from build123d import *

# Parameters (mm, degrees)
SKETCH3_W           = 40
SKETCH3_H           = 40
SKETCH3_R           = 5
SKETCH3_R_2         = 2.4
BOSS_EXTRUDE2_DEPTH = 3
BOSS_EXTRUDE3_DEPTH = 8
SKETCH6_W           = 2
SKETCH6_H           = 5
BOSS_EXTRUDE5_DEPTH = 5
SKETCH7_W           = 40
SKETCH7_H           = 6.5
CUT_EXTRUDE1_DEPTH  = 3
SKETCH8_W           = 40
SKETCH8_H           = 6.5
CUT_EXTRUDE2_DEPTH  = 3
CUT_EXTRUDE3_START  = -1
SKETCH5_W           = 5
SKETCH5_H           = 0.5
CUT_EXTRUDE3_DEPTH  = 6


with BuildPart() as part:
    # Sketch3 → Boss-Extrude2 (new body)
    with BuildSketch(Plane(origin=(0, 0, 0), x_dir=(1, 0, 0), z_dir=(0, 1, 0))):
        Rectangle(SKETCH3_W, SKETCH3_H)
        Circle(SKETCH3_R, mode=Mode.SUBTRACT)
        Circle(SKETCH3_R)
        Circle(SKETCH3_R_2, mode=Mode.SUBTRACT)
    extrude(amount=-BOSS_EXTRUDE2_DEPTH)

    # Sketch4 → Boss-Extrude3 (add)
    with BuildSketch(Plane.XZ.offset(3)):
        Polygon((20, -11.5), (0, -11.5), (-20, -11.5), (-20, -13.5), (20, -13.5), align=None)
        Polygon((-20, 11.5), (0, 11.5), (20, 11.5), (20, 13.5), (-20, 13.5), align=None)
    extrude(amount=BOSS_EXTRUDE3_DEPTH)

    # Sketch6 → Boss-Extrude5 (add)
    with BuildSketch(Plane.XZ.offset(3)):
        with Locations((19, 9)):
            Rectangle(SKETCH6_W, SKETCH6_H)
        with Locations((19, -9)):
            Rectangle(SKETCH6_W, SKETCH6_H)
        with Locations((-19, -9)):
            Rectangle(SKETCH6_W, SKETCH6_H)
        with Locations((-19, 9)):
            Rectangle(SKETCH6_W, SKETCH6_H)
    extrude(amount=BOSS_EXTRUDE5_DEPTH)

    # Sketch7 → Cut-Extrude1 (cut)
    with BuildSketch(Plane(origin=(0, -3, 0), x_dir=(-1, 0, 0), z_dir=(0, -1, 0))):
        with Locations((0, -16.75)):
            Rectangle(SKETCH7_W, SKETCH7_H)
    extrude(amount=-CUT_EXTRUDE1_DEPTH, mode=Mode.SUBTRACT)

    # Sketch8 → Cut-Extrude2 (cut)
    with BuildSketch(Plane.XZ.offset(3)):
        with Locations((0, -16.75)):
            Rectangle(SKETCH8_W, SKETCH8_H)
    extrude(amount=-CUT_EXTRUDE2_DEPTH, mode=Mode.SUBTRACT)

    # Sketch5 → Cut-Extrude3 (cut)
    with BuildSketch(Plane.XY.offset(-11.5).offset(CUT_EXTRUDE3_START)):
        Polygon((19, -7.5), (0, -7.5), (0, -8), (5, -8), (5, -8.5), (19, -8.5), align=None)
        Polygon((0, -8), (0, -7.5), (-19, -7.5), (-19, -8.5), (-5, -8.5), (-5, -8), align=None)
        with Locations((-2.5, -8.25)):
            Rectangle(SKETCH5_W, SKETCH5_H)
        with Locations((2.5, -8.25)):
            Rectangle(SKETCH5_W, SKETCH5_H)
    cut_extrude3 = extrude(amount=CUT_EXTRUDE3_DEPTH, mode=Mode.SUBTRACT)

    # Mirror2: Cut-Extrude3 across plane
    add(cut_extrude3.mirror(Plane.XY), mode=Mode.SUBTRACT)


solid = part.part
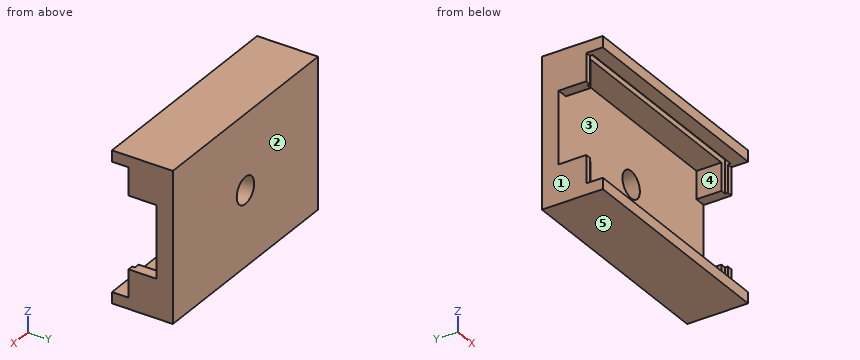
Read the model definition and answer for the solid it produces. Units are mm, in the model's axes. Face numbers are marked on the shaded views. A direction names the side the tool comes from. Coordinates: 2 decimals unless noted, no trailing zeros. Order: outer loops, then holes, each group sorted by start corner. A loop starts at its lowest first (then second) coordinate and runs counter-clockwise, first axis right, second up. Notation, with made-up numbers: (65.5, 70.5) -> (82.5, 70.5) arc R20 ccw to (82.5, 97.5) -> close; hole circle Ø8 at (71, 24). An arc over 180 degrees is marked (long way). Answer as a JSON object with one key per item and string values.
1) A cutting plane is placed at B-B, the plane x = 0. Determine the outline of the cut face in (y, z), plus the area to 3 significant figures.
Model answer:
{"outline": "(-11, -13.5) -> (0, -13.5) -> (0, -2.4) -> (-3, -2.4) -> (-3, -11.5) -> (-7.5, -11.5) -> (-7.5, -12.5) -> (-8.5, -12.5) -> (-8.5, -11.5) -> (-11, -11.5) -> close; (-11, 11.5) -> (-8.5, 11.5) -> (-8.5, 12.5) -> (-7.5, 12.5) -> (-7.5, 11.5) -> (-3, 11.5) -> (-3, 2.4) -> (0, 2.4) -> (0, 13.5) -> (-11, 13.5) -> close", "area": "96.6 mm²"}
2) A cutting plane is placed at A-A, the plane y = -4.5. Determine the outline of the cut face in (x, z), plus the area to 3 significant figures.
Model answer:
{"outline": "(-20, -13.5) -> (20, -13.5) -> (20, -6.5) -> (18, -6.5) -> (18, -11.5) -> (-18, -11.5) -> (-18, -6.5) -> (-20, -6.5) -> close; (-20, 6.5) -> (-18, 6.5) -> (-18, 11.5) -> (18, 11.5) -> (18, 6.5) -> (20, 6.5) -> (20, 13.5) -> (-20, 13.5) -> close", "area": "200 mm²"}
3) A cutting plane is placed at C-C, the plane z = 0. Determine the outline of the cut face in (x, y), plus the area to 3 significant figures.
Model answer:
{"outline": "(-20, -3) -> (-2.4, -3) -> (-2.4, 0) -> (-20, 0) -> close; (2.4, -3) -> (20, -3) -> (20, 0) -> (2.4, 0) -> close", "area": "106 mm²"}
4) The mould has two halves that part along X. Classify the marked faces 1, 2 and 3: released by +X, released by -X, zero draft, split by the parting line, or undercut.
Model answer:
{"face 1": "released by -X", "face 2": "zero draft", "face 3": "undercut"}
5) A tool of negligible diameter and unlimited length cuts with its end or side. For the marked faces 4 and 5, from which of +Z, -Z, +X, -X, +Y, -Y can it reach the whole face along a straight path? Write none if from no direction.
Model answer:
{"face 4": "-Y", "face 5": "-Z, +X, -X, +Y, -Y"}
6) A cutting plane is placed at D-D, the plane y = -1.25. Determine the outline of the cut face in (x, z).
Model answer:
{"outline": "(-20, -13.5) -> (20, -13.5) -> (20, 13.5) -> (-20, 13.5) -> close; hole circle Ø4.8 at (0, 0)"}
7) Consider line 1 along Y through (x, z) = (-11.5, 11.75); line 2 along X through (y, z) = (-1.8, 0); line 3 along Z through (x, y) = (0, -1.75). Determine where each line is inside the solid, lowest interval first. Write a range as from..to.
Model answer:
{"line 1": "y = -11..-8.5, -7.5..0", "line 2": "x = -20..-2.4, 2.4..20", "line 3": "z = -13.5..-2.4, 2.4..13.5"}
8) Each of these flat-tipped pins is pushed along its axis until it touches: pin 1 (0.8 mm diameter, centred on x = 19.5, z = -8, fed in from -Y); pin 2 (1.8 mm diameter, centred on x = 7, z = 8, fed in from -Y). Where does it stop, or does it pass through?
Model answer:
{"pin 1": "stops at y = -8", "pin 2": "stops at y = -3"}
